Could you check a few things on this model? Use its own coordinates, in mm. A direction names the side the tool comes from. Coordinates: 2 decimals unless noted, no trailing zeros. Loops run counter-clockwise (first coordinate to the right, second up) from the corner with the lowest first, then second, coordinate; pieces in that order, holes last. Notation, with made-up numbers: M 1.25,86 L 57.25,86 A19 ccw 57.25,123 Z; hole C -15.75,64 d3. An arc over 180 degrees is marked long. Write each question's results on one line, items separated by ' | '.
```python
from build123d import *

# Parameters (mm, degrees)
ESQUISSE1_W             = 44
ESQUISSE1_H             = 42
ESQUISSE1_R             = 4.065
BOSS_EXTRU_1_DEPTH      = 12
ESQUISSE2_W             = 5.9
ESQUISSE2_H             = 42
ESQUISSE2_W_2           = 11.75
ESQUISSE2_R             = 4.065
BOSS_EXTRU_2_DEPTH      = 19
ESQUISSE3_W             = 5.9
ESQUISSE3_H             = 42
ENL_V_MAT_EXTRU_1_DEPTH = 16
CONG_1_R                = 2
CONG_2_R                = 1
CONG_3_R                = 1


with BuildPart() as part:
    # Esquisse1 → Boss.-Extru.1 (new body)
    with BuildSketch(Plane(origin=(0, 0, 0), x_dir=(1, 0, 0), z_dir=(0, 1, 0))):
        Rectangle(ESQUISSE1_W, ESQUISSE1_H)
        with Locations(Location((-15.1, 11.875, 0), (0, 0, 270))):
            Circle(ESQUISSE1_R, mode=Mode.SUBTRACT)
        with Locations(Location((15.1, 11.875, 0), (0, 0, 90))):
            Circle(ESQUISSE1_R, mode=Mode.SUBTRACT)
        with Locations(Location((15.1, -11.875, 0), (0, 0, 270))):
            Circle(ESQUISSE1_R, mode=Mode.SUBTRACT)
        with Locations(Location((-15.1, -11.875, 0), (0, 0, 90))):
            Circle(ESQUISSE1_R, mode=Mode.SUBTRACT)
    extrude(amount=BOSS_EXTRU_1_DEPTH)

    # Esquisse2 → Boss.-Extru.2 (add)
    # profile 1 of 3: a face of its own
    with BuildSketch(Plane(origin=(0, 12, 0), x_dir=(1, 0, 0), z_dir=(0, 1, 0))):
        Rectangle(ESQUISSE2_W, ESQUISSE2_H)
    # profile 2 of 3: a face of its own
    with BuildSketch(Plane(origin=(0, 12, 0), x_dir=(1, 0, 0), z_dir=(0, 1, 0))):
        with Locations((-16.125, 0)):
            Rectangle(ESQUISSE2_W_2, ESQUISSE2_H)
        with Locations(Location((-15.1, -11.875, 0), (0, 0, 90))):
            Circle(ESQUISSE2_R, mode=Mode.SUBTRACT)
        with Locations(Location((-15.1, 11.875, 0), (0, 0, 270))):
            Circle(ESQUISSE2_R, mode=Mode.SUBTRACT)
    # profile 3 of 3: a face of its own
    with BuildSketch(Plane(origin=(0, 12, 0), x_dir=(1, 0, 0), z_dir=(0, 1, 0))):
        with Locations((16.125, 0)):
            Rectangle(ESQUISSE2_W_2, ESQUISSE2_H)
        with Locations(Location((15.1, 11.875, 0), (0, 0, 90))):
            Circle(ESQUISSE2_R, mode=Mode.SUBTRACT)
        with Locations(Location((15.1, -11.875, 0), (0, 0, 270))):
            Circle(ESQUISSE2_R, mode=Mode.SUBTRACT)
    extrude(amount=BOSS_EXTRU_2_DEPTH)

    # Esquisse3 → Enlèv. mat.-Extru.1 (cut)
    with BuildSketch(Plane(origin=(0, 31, 0), x_dir=(1, 0, 0), z_dir=(0, 1, 0))):
        Rectangle(ESQUISSE3_W, ESQUISSE3_H)
    extrude(amount=-ENL_V_MAT_EXTRU_1_DEPTH, mode=Mode.SUBTRACT)

    # Congé1
    cong_1_edges = [part.edges().sort_by_distance(p)[0] for p in [
        (-22, 15.5, -21),
        (22, 15.5, -21),
        (22, 15.5, 21),
        (-22, 15.5, 21),
    ]]
    fillet(cong_1_edges, radius=CONG_1_R)

    # Congé2
    cong_2_edges = [part.edges().sort_by_distance(p)[0] for p in [
        (-10.25, 21.5, 21),
        (-10.25, 21.5, -21),
        (10.25, 21.5, -21),
        (10.25, 21.5, 21),
        (-2.95, 13.5, 21),
        (-2.95, 13.5, -21),
        (2.95, 13.5, -21),
        (2.95, 13.5, 21),
    ]]
    fillet(cong_2_edges, radius=CONG_2_R)

    # Congé3
    # the kernel refuses this fillet: 1 mm, written as the material it adds along each edge
    with BuildSketch(Plane(origin=(10.25, 12, -20), x_dir=(0, 1, 0), z_dir=(0, 0, 1))) as cong_3_piece_1:
        with BuildLine():
            CenterArc((CONG_3_R, CONG_3_R), CONG_3_R, 180, 90)
            Line((0, CONG_3_R), (0, 0))
            Line((0, 0), (CONG_3_R, 0))
        make_face()
    extrude(amount=40)
    with BuildSketch(Plane(origin=(-10.25, 12, -20), x_dir=(0, 1, 0), z_dir=(0, 0, 1))) as cong_3_piece_2:
        with BuildLine():
            CenterArc((CONG_3_R, -CONG_3_R), CONG_3_R, 90, 90)
            Line((0, -CONG_3_R), (0, 0))
            Line((0, 0), (CONG_3_R, 0))
        make_face()
    extrude(amount=40)
    with BuildSketch(Plane(origin=(11.25, 12, -20), x_dir=(0.5976672776328271, 0, 0.8017442392976486), z_dir=(-0.8017442392976486, 0, 0.5976672776328271))) as cong_3_piece_3_section:
        with BuildLine():
            CenterArc((1 + CONG_3_R, CONG_3_R), CONG_3_R, 180, 90)
            Line((1, CONG_3_R), (1, 0))
            Line((1, 0), (1 + CONG_3_R, 0))
        make_face()
    cong_3_piece_3 = revolve(axis=Axis((11.25, 12, -20), (0, 1, 0)), revolution_arc=233.296989237, mode=Mode.PRIVATE)
    cong_3_piece_3 = split(cong_3_piece_3, bisect_by=Plane(origin=(10.500061043, 12.311628317, -21), z_dir=(0, 0, 1)), keep=Keep.TOP, mode=Mode.PRIVATE)
    add(cong_3_piece_3)
    with BuildSketch(Plane(origin=(11.25, 12, 20), x_dir=(-1, 0, 0), z_dir=(0, 0, -1))) as cong_3_piece_4_section:
        with BuildLine():
            CenterArc((1 + CONG_3_R, CONG_3_R), CONG_3_R, 180, 90)
            Line((1 + CONG_3_R, 0), (1, 0))
            Line((1, 0), (1, CONG_3_R))
        make_face()
    cong_3_piece_4 = revolve(axis=Axis((11.25, 12, 20), (0, 1, 0)), revolution_arc=233.296989237, mode=Mode.PRIVATE)
    cong_3_piece_4 = split(cong_3_piece_4, bisect_by=Plane(origin=(10.500061142, 12.311628426, 21), z_dir=(0, 0, -1)), keep=Keep.TOP, mode=Mode.PRIVATE)
    add(cong_3_piece_4)
    with BuildSketch(Plane(origin=(-11.25, 12, -20), x_dir=(-0.5976672776328282, 0, 0.8017442392976477), z_dir=(0.8017442392976477, 0, 0.5976672776328282))) as cong_3_piece_5_section:
        with BuildLine():
            CenterArc((1 + CONG_3_R, -CONG_3_R), CONG_3_R, 90, 90)
            Line((1 + CONG_3_R, 0), (1, 0))
            Line((1, 0), (1, -CONG_3_R))
        make_face()
    cong_3_piece_5 = revolve(axis=Axis((-11.25, 12, -20), (0, -1, 0)), revolution_arc=233.296989237, mode=Mode.PRIVATE)
    cong_3_piece_5 = split(cong_3_piece_5, bisect_by=Plane(origin=(-10.500061216, 12.311628717, -21), z_dir=(0, 0, 1)), keep=Keep.TOP, mode=Mode.PRIVATE)
    add(cong_3_piece_5)
    with BuildSketch(Plane(origin=(-11.25, 12, 20), x_dir=(1, 0, 0), z_dir=(0, 0, -1))) as cong_3_piece_6_section:
        with BuildLine():
            CenterArc((1 + CONG_3_R, -CONG_3_R), CONG_3_R, 90, 90)
            Line((1 + CONG_3_R, 0), (1, 0))
            Line((1, 0), (1, -CONG_3_R))
        make_face()
    cong_3_piece_6 = revolve(axis=Axis((-11.25, 12, 20), (0, -1, 0)), revolution_arc=233.296989237, mode=Mode.PRIVATE)
    cong_3_piece_6 = split(cong_3_piece_6, bisect_by=Plane(origin=(-10.500060984, 12.311628017, 21), z_dir=(0, 0, -1)), keep=Keep.TOP, mode=Mode.PRIVATE)
    add(cong_3_piece_6)


solid = part.part
```
(1) Will these pins go through, and if not, where does the flat tip stop? P1, Ø2.5, axis at x = -4.5, z = 0, coming from the +Y side; P2, Ø3, axis at x = -1, z = 11, coming from the +Y side.
Reported:
P1: stops at y = 12 | P2: stops at y = 15
(2) Imagine slicing it at D-D, the plane y = 4. List the corners of the cut face in (x, z) for me (3 decimals), and give its area (3 significant figures).
Reported:
outline: M -22,-19 A2 ccw -20,-21 L 20,-21 A2 ccw 22,-19 L 22,19 A2 ccw 20,21 L -20,21 A2 ccw -22,19 Z; hole C -15.1,-11.875 d8.13; hole C -15.1,11.875 d8.13; hole C 15.1,-11.875 d8.13; hole C 15.1,11.875 d8.13 | area: 1,640 mm2
(3) Imagine slicing it at B-B, the plane x = -15.1. List the corners of the cut face in (y, z) for me.
Reported:
outline: M 0,-21 L 31,-21 L 31,-15.94 L 0,-15.94 Z; M 0,-7.81 L 31,-7.81 L 31,7.81 L 0,7.81 Z; M 0,15.94 L 31,15.94 L 31,21 L 0,21 Z
(4) If we mould it in two halves opening along Z, with no side actions, what happens to faces 1 (the cylindrical face through (-21.43, 15.28, -20.4)), 2 (the cylindrical face through (21.4, 15.72, 20.43)), 3 (the flat face through (-16, 31, 0)), 4 (the cylindrical face through (16.321, 15.283, 15.752))? For each: released by +Z, released by -Z, zero draft, split by the parting line, or undercut.
Reported:
face 1: released by -Z | face 2: released by +Z | face 3: zero draft | face 4: undercut
(5) Imagine slicing it at A-A, the plane y = 28.5. List the corners of the cut face in (x, z) for me (3 decimals), and give its area (3 significant figures).
Reported:
outline: M -22,-19 A2 ccw -20,-21 L -11.25,-21 A1 ccw -10.25,-20 L -10.25,20 A1 ccw -11.25,21 L -20,21 A2 ccw -22,19 Z; M 10.25,-20 A1 ccw 11.25,-21 L 20,-21 A2 ccw 22,-19 L 22,19 A2 ccw 20,21 L 11.25,21 A1 ccw 10.25,20 Z; hole C -15.1,-11.875 d8.13; hole C -15.1,11.875 d8.13; hole C 15.1,-11.875 d8.13; hole C 15.1,11.875 d8.13 | area: 775 mm2
(6) Please list where these lines run through material, in increasing order: probe 1 along Z at (x, y) = (-15, 20); probe 2 along Z at (x, y) = (11.5, 29.5); probe 3 along X at (y, z) = (4, -12). Write a range as from..to.
Reported:
probe 1: z = -21..-15.94, -7.81..7.81, 15.94..21 | probe 2: z = -21..-13.76, -9.99..9.99, 13.76..21 | probe 3: x = -22..-19.16, -11.04..11.04, 19.16..22
(7) Which directions (+Z, -Z, +X, -X, +Y, -Y) give clear straight access to the entire face, cutting with the end or side of a thin tool? Please do faces 5 (the flat face through (2.95, 13, 0)), 6 (the flat face through (0, 12, 21)).
Reported:
face 5: +Z, -Z, +Y | face 6: +Z, +X, -X, +Y, -Y
(8) Imagine slicing it at C-C, the plane z = 14.5. List the corners of the cut face in (x, y) for me, and give its area (3 significant figures).
Reported:
outline: M -22,0 L -18.2,0 L -18.2,31 L -22,31 Z; M -12,0 L 12,0 L 12,31 L 10.25,31 L 10.25,13 A1 cw 9.25,12 L 2.95,12 L 2.95,15 L -2.95,15 L -2.95,12 L -9.25,12 A1 cw -10.25,13 L -10.25,31 L -12,31 Z; M 18.2,0 L 22,0 L 22,31 L 18.2,31 Z | area: 608 mm2
